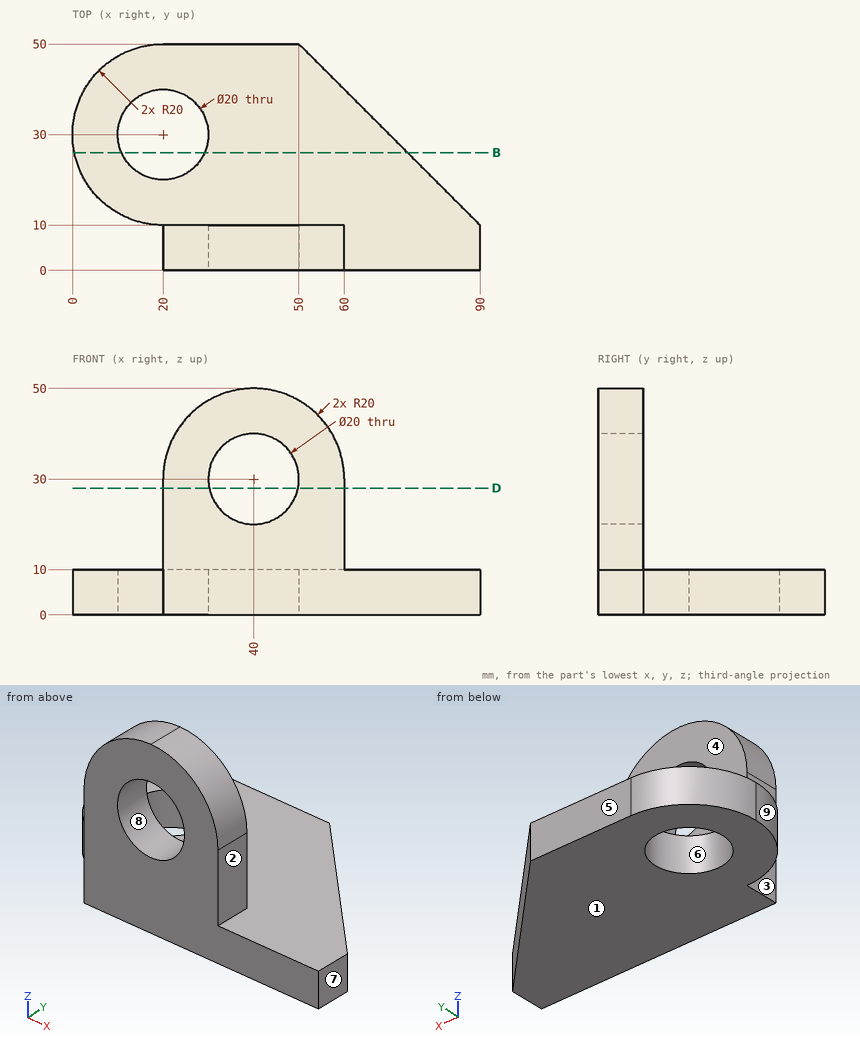
Answer from the drawing. Dimensions are ordinates in mm from the lowest x, y and z of the part. A direction names the side the tool comes from. Coordinates: 2 decimals unless noted, no trailing zeros. Write each loop counter-clockwise with the first axis right and the second up, starting at its lowest first coordinate (ties: lowest second). Pieces come first, ordered by that corner, then holes. Notation, with made-up numbers: (36.25, -38) - (95.25, -38) arc R21 cw to (95.25, -26) - close; hole circle Ø7 at (52.5, 38.5). An arc over 180 degrees is marked (long way). Answer as CSV lines item,"result".
1. Find section B-B (y = 26). Give the vertices of the cut face in (x, z) (3 decimals), plus the area to 3 significant figures.
Computed values:
outline,"(0.404, 0) - (10.835, 0) - (10.835, 10) - (0.404, 10) - close; (29.165, 0) - (74, 0) - (74, 10) - (29.165, 10) - close"
area,"553 mm²"
2. A tool of negligible diameter and unlimited length cuts with its end or side. For the marked faces 1, 2, 3, 4 and 5, from which of +Z, -Z, +X, -X, +Y, -Y can it reach the whole face along a straight path? Write none if from no direction.
Computed values:
face 1,"-Z, +X, -X, +Y, -Y"
face 2,"+Z, +X, +Y, -Y"
face 3,"+Z, -Z, -X, -Y"
face 4,"+Z, +X, -X, +Y"
face 5,"+Z, -Z, +X, -X, +Y"
3. Straight lines are drawn through the part: line 1 (Z direction, x = 40, y = 3.5); line 2 (Y direction, x = 57, z = 29). For each, find the intervals that lie inside material, in ascending order. Write a range as [from, to].
Computed values:
line 1,"z = [0, 20], [40, 50]"
line 2,"y = [0, 10]"
4. Find section D-D (z = 28). Give the vertices of the cut face in (x, y), plus the area to 3 significant figures.
Computed values:
outline,"(20, 0) - (30.2, 0) - (30.2, 10) - (20, 10) - close; (49.8, 0) - (60, 0) - (60, 10) - (49.8, 10) - close"
area,"204 mm²"
5. Given P1, Ø8, axis at y = 5, z = 21, coming from the +X side; P2, Ø10, axis at x = 78.5, z = 12.5, coming from the +Y side; P3, Ø5, axis at x = 44, z = 41, coming from the +Y side, each flat-ended and moving along its own axis, determine where each tip first touches the part or whether it passes through.
Computed values:
P1,"stops at x = 60"
P2,"stops at y = 25.83"
P3,"stops at y = 10"
6. Determine the mould class of the marked faces 6, 7, 8 and 9 for opening direction X: +X half, -X half, draft (parallel to the pull), parting line (faces both ways), or undercut.
Computed values:
face 6,"undercut"
face 7,"+X half"
face 8,"undercut"
face 9,"-X half"
